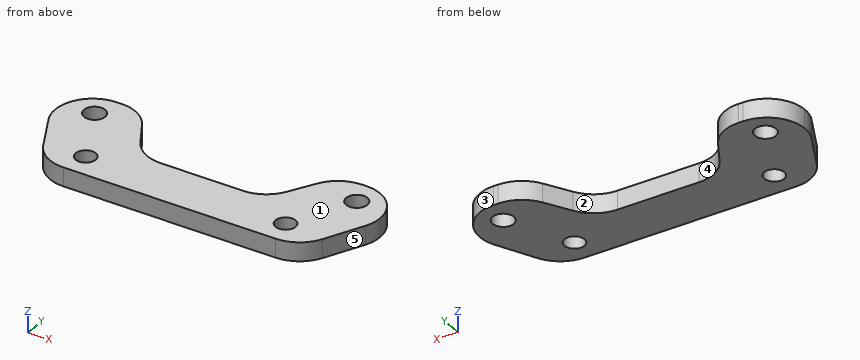
Autodesk Inventor part; units mm, degrees
ref_plane "YZ Plane" through (0, 0, 0) normal (1, 0, 0) x (0, 1, 0)
ref_plane "XZ Plane" through (0, 0, 0) normal (0, 1, 0) x (-1, 0, 0)
ref_plane "XY Plane" through (0, 0, 0) normal (0, 0, 1) x (1, 0, 0)
sketch "スケッチ2" plane through (0, 0, 0) normal (0, 0, 1) x (1, 0, 0)
  line L0 (0, 0) -> (26, 0)
  line L1 (26, 0) -> (26, 33)
  line L2 (26, 33) -> (0, 33)
  line L3 (0, 33) -> (0, 0)
  line L4 (0, 0) -> (26, 0)
  line L5 (26, 0) -> (26, 24)
  line L6 (26, 24) -> (0, 24) construction
  line L7 (0, 24) -> (0, 0)
  circle A0 centre (13, 24) radius 13
  circle A1 centre (13, 24) radius 6.25
  line L8 (26, 0) -> (0, 0)
  line L9 (0, 0) -> (0, -4)
  line L10 (0, -4) -> (26, -4)
  line L11 (26, -4) -> (26, 0)
  circle A2 centre (21, -2) radius 0.8
  circle A3 centre (5, -2) radius 0.8
  point P0 (22.3808, 33)
  point P1 (3.6192, 33)
  point P2 (26, -2)
  dimension "d0" = 26
  dimension "d1" = 33
  dimension "d2" = 24
  dimension "d3" = 12.5
  dimension "d8" = 4
  dimension "d9" = 1.6
  dimension "d10" = 1.6
  dimension "d12" = 5
  dimension "d13" = 5
extrude "押し出し1" add sketch "スケッチ2" along normal blind 1.5 contours L3 A0 L1 L0 | L0 L11 L10 L9 | A0 L2 picked at (12.7489, 32.0681)
sketch "スケッチ3" plane through (0, 0, 0) normal (0, 0, -1) x (-1, 0, 0)
  circle A0 centre (-2.5, 24) radius 0.85
  circle A1 centre (-23.5, 24) radius 0.85
  circle A2 centre (-23.5, 3) radius 0.85
  circle A3 centre (-2.5, 3) radius 0.85
  point P0 (0, 0)
extrude "押し出し2" cut sketch "スケッチ3" against normal through all
fillet "フィレット1" radius 3 4 edges at (22.3808, 33, 0.75) (3.6192, 33, 0.75) (26, -4, 0.75) (0, -4, 0.75)
sketch "スケッチ4" plane through (0, 0, 1.5) normal (0, 0, 1) x (1, 0, 0)
  line L0 (0, 24) -> (0, -1)
  line L1 (0, 5) -> (26, 5)
  line L2 (26, 5) -> (26, 33)
  line L3 (26, 33) -> (0, 33)
  line L4 (0, 33) -> (0, 5)
  line L5 (21, 33) -> (5, 33)
  line L6 (26, -1) -> (26, 24)
  circle A0 centre (2.5, 3) radius 0.85
  line L7 (5.1132, 5) -> (8, 0)
  line L8 (8, 0) -> (18, 0)
  line L9 (18, 0) -> (20.8868, 5)
  line L10 (0, 1.2918) -> (2.6459, -4)
  line L11 (3, -4) -> (23, -4)
  line L12 (26, 1.2918) -> (23.3541, -4)
  arc A1 (0, -1) -> (3, -4) centre (3, -1) ccw
  arc A2 (23, -4) -> (26, -1) centre (23, -1) ccw
  line L13 (2.5, 3) -> (5, -2)
  circle A3 centre (5, -2) radius 0.8
  circle A4 centre (21, -2) radius 0.8
  circle A5 centre (23.5, 3) radius 0.85
  line L14 (23.5, 3) -> (21, -2)
  point P0 (0, 0)
  point P1 (13, 0)
  point P2 (13, 5)
  point P3 (23.3653, -3.9777)
  point P4 (2.6347, -3.9777)
  dimension "d15" = 2
  dimension "d16" = 10
  dimension "d17" = 5
  dimension "d18" = 120
  dimension "d19" = 120
  dimension "d24" = 3
  dimension "d25" = 3
extrude "切り取り1" cut sketch "スケッチ4" against normal blind 3.048 contours L4 L3 L2 L1 L0 | L1 L9 L8 L7
extrude "押し出し3" cut sketch "スケッチ4" against normal through all contours L10 A1 L0 | L6 A2 L12
fillet "フィレット3" radius 3 10 edges at (5.1132, 5, 0.75) (0, 5, 0.75) (8, 0, 0.75) (20.8868, 5, 0.75) (26, 5, 0.75) (26, 1.2918, 0.75) (18, 0, 0.75) (0, 1.2918, 0.75) (2.6347, -3.9777, 0.75) (23.3653, -3.9777, 0.75)
equation "\"d13\" = d12"
equation "\"d19\" = d18"
equation "\"d25\" = d24"
equation "\"d21\" = Thickness"
equation "\"BendRadius\" = Thickness"
equation "\"BendReliefWidth\" = Thickness"
equation "\"BendReliefDepth\" = 0.5 * Thickness"
equation "\"CornerReliefSize\" = 4 * Thickness"
equation "\"MinimumRemnant\" = 2 * Thickness"
equation "\"TransitionRadius\" = BendRadius"
equation "\"JacobiRadiusSize\" = BendRadius"
equation "\"GapSize\" = Thickness"
equation "\"d20\" = Thickness"
properties part number "upper_arm" material "アルミニウム 6061"
Verification items for the finished model (mm, model axes). Face numbers are marked on the shaded views. A direction names the side the tool comes from. Coordinates: 2 decimals unless noted, no trailing zeros. Loops run counter-clockwise (first coordinate to the right, second up) from the corner with the lowest first, then second, coordinate; pieces in that order, holes last. Notation, with made-up numbers: (35, -25) -> (63, -25) arc R19 ccw to (63, -21) -> close; hole circle Ø4 at (6.25, 82). An arc over 180 degrees is marked (long way). Answer in a Markdown table with one row per item. Add a question column.
1. Section check C-C, the plane x = 5. Enter the section's corners in (y, z), then the cut area to 3 significant figures.
2. Material ranges on probe 1 along X at (y, z) = (2.5, 0.75); probe 2 along Y at (x, z) = (23.75, 0.7); probe 3 along Y at (x, z) = (5, 0.95), recorded low to high. Write a range as [from, to].
3. Section check B-B, the plane y = 3. Enter the section's corners in (x, z).
4. Draft check along X on the marked faces 1, 2 and 3. Enter one of: +X half, -X half, draft (parallel to the pull), parting line (faces both ways), or undercut.
5. Section check A-A, the plane z = 1. Give the number of separate pieces and of enclosed holes in the cut face, then the cut area to 3 significant figures.
6. Depth check by flat-ended pin: P1, Ø2, axis at x = 2.5, y = 3, coming from the -Z side. Enter the tip coordinate at first touch or a pass-through.
7. Access from +Z, -Z, +X, -X, +Y, -Y to the whole of each face (thin tool, end or side, straight path). Record for the marked faces 4 and 5.
8. Section check D-D, the plane y = -2. Enter the section's corners in (x, z).
Derived:
| question | item | result |
|---|---|---|
| 1 | outline | (-4, 0) -> (-2.8, 0) -> (-2.8, 1.5) -> (-4, 1.5) -> close; (-1.2, 0) -> (4.53, 0) -> (4.53, 1.5) -> (-1.2, 1.5) -> close |
| 1 | area | 10.4 mm² |
| 2 | probe 1 | x = [0.04, 1.81], [3.19, 6.56], [19.44, 22.81], [24.19, 25.96] |
| 2 | probe 2 | y = [-2.98, 2.19], [3.81, 4.9] |
| 2 | probe 3 | y = [-4, -2.8], [-1.2, 4.53] |
| 3 | outline | (0.17, 0) -> (1.65, 0) -> (1.65, 1.5) -> (0.17, 1.5) -> close; (3.35, 0) -> (6.27, 0) -> (6.27, 1.5) -> (3.35, 1.5) -> close; (19.73, 0) -> (22.65, 0) -> (22.65, 1.5) -> (19.73, 1.5) -> close; (24.35, 0) -> (25.83, 0) -> (25.83, 1.5) -> (24.35, 1.5) -> close |
| 4 | face 1 | draft |
| 4 | face 2 | undercut |
| 4 | face 3 | +X half |
| 5 | separate pieces | 1 |
| 5 | enclosed holes | 4 |
| 5 | area | 142 mm² |
| 6 | P1 | stops at z = 0 |
| 7 | face 4 | +Z, -Z, +Y |
| 7 | face 5 | +Z, -Z, +X, -Y |
| 8 | outline | (1.65, 0) -> (4.2, 0) -> (4.2, 1.5) -> (1.65, 1.5) -> close; (5.8, 0) -> (20.2, 0) -> (20.2, 1.5) -> (5.8, 1.5) -> close; (21.8, 0) -> (24.35, 0) -> (24.35, 1.5) -> (21.8, 1.5) -> close |
